CAD build for the part. Positions are in the model's coordinates, mm. Give positions to 0.01 mm unless a question says otherwise; leave off trailing zeros. Loops run counter-clockwise (first coordinate to the right, second up) from the corner with the lowest first, then second, coordinate; pieces in that order, holes last.
```python
from build123d import *

# Parameters (mm, degrees)
SKETCH1_R                = 1.5
BOSS_EXTRUDE2_DEPTH      = 1.7
BOSS_EXTRUDE3_DEPTH      = 7.3
BOSS_EXTRUDE3_DEPTH_BACK = 4.1
SKETCH2_W                = 16.43
SKETCH2_H                = 15.24


with BuildPart() as part:
    # Sketch1 → Boss-Extrude2 (new body)
    with BuildSketch(Plane(origin=(0, 0, 0), x_dir=(0, 0, -1), z_dir=(1, 0, 0))):
        with BuildLine():
            Line((-33, 66.67), (33, 66.67))
            ThreePointArc((33, 66.67), (34.414213562, 66.084213562), (35, 64.67))
            Line((35, 64.67), (35, -64.67))
            ThreePointArc((35, -64.67), (34.414213562, -66.084213562), (33, -66.67))
            Line((33, -66.67), (-33, -66.67))
            ThreePointArc((-33, -66.67), (-34.414213562, -66.084213562), (-35, -64.67))
            Line((-35, -64.67), (-35, 64.67))
            ThreePointArc((-35, 64.67), (-34.414213562, 66.084213562), (-33, 66.67))
        make_face()
        with Locations((-22.86, -37.46)):
            Circle(SKETCH1_R, mode=Mode.SUBTRACT)
        with Locations((22.86, -37.46)):
            Circle(SKETCH1_R, mode=Mode.SUBTRACT)
        with Locations((-24.13, 37.63)):
            Circle(SKETCH1_R, mode=Mode.SUBTRACT)
        with Locations((24.13, 37.63)):
            Circle(SKETCH1_R, mode=Mode.SUBTRACT)
        with Locations((8.89, -13.17)):
            Circle(SKETCH1_R, mode=Mode.SUBTRACT)
    extrude(amount=BOSS_EXTRUDE2_DEPTH)

    # Sketch2 → Boss-Extrude3 (add, two sides: drawn at the far end of the back side and taken through both)
    with BuildSketch(Plane(origin=(1.7, 0, 0), x_dir=(0, 0, -1), z_dir=(1, 0, 0)).offset(-BOSS_EXTRUDE3_DEPTH_BACK)):
        with Locations((9.225, -61.59)):
            Rectangle(SKETCH2_W, SKETCH2_H)
    extrude(amount=BOSS_EXTRUDE3_DEPTH + BOSS_EXTRUDE3_DEPTH_BACK)


solid = part.part
```
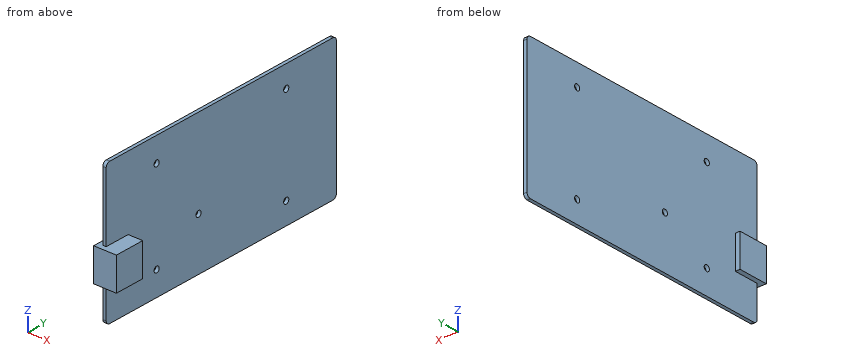
1. Probe line 1 along Y through (x, z) = (0.8, -22.86); line 2 along Y through (x, z) = (1.35, -24.13); line 3 along X through (y, z) = (39.5, 27). List the from-to ranges inside material, lowest first.
Responses:
line 1: y = -66.67 to -38.96, -35.96 to 36.83, 38.43 to 66.67
line 2: y = -66.67 to -38.26, -36.66 to 36.13, 39.13 to 66.67
line 3: x = 0 to 1.7
2. Saw through at C-C, the plane y = -13.17. List the corners of the cut face in (x, z).
Responses:
outline: (0, -35) - (1.7, -35) - (1.7, -10.39) - (0, -10.39) - close; (0, -7.39) - (1.7, -7.39) - (1.7, 35) - (0, 35) - close
3. Saw through at D-D, the plane y = -59.5. List the corners of the cut face in (x, z), and give its area (3 significant figures).
Responses:
outline: (-2.4, -17.44) - (0, -17.44) - (0, -35) - (1.7, -35) - (1.7, -17.44) - (9, -17.44) - (9, -1.01) - (1.7, -1.01) - (1.7, 35) - (0, 35) - (0, -1.01) - (-2.4, -1.01) - close
area: 278 mm2
4. Saw through at A-A, the plane y = -37.46. List the corners of the cut face in (x, z), and give its area (3 significant figures).
Responses:
outline: (0, -35) - (1.7, -35) - (1.7, -24.36) - (0, -24.36) - close; (0, -21.36) - (1.7, -21.36) - (1.7, 21.36) - (0, 21.36) - close; (0, 24.36) - (1.7, 24.36) - (1.7, 35) - (0, 35) - close
area: 109 mm2
5. Drop flat-ended pins along their axis: pin 1 (1.9 mm diameter, centred on x = 0.5, z = -24, fed in from -Y); pin 2 (5 mm diameter, centred on y = -37.46, z = -22.86, fed in from +X); pin 3 (1.8 mm diameter, centred on y = 37.63, z = 24.13, fed in from +X); pin 4 (2 mm diameter, centred on x = 6, z = -10, fed in from +Y). Give the stop position or say it passes through.
Responses:
pin 1: stops at y = -66.67
pin 2: stops at x = 1.7
pin 3: passes through
pin 4: stops at y = -53.97
6. Saw through at B-B, the plane z = -8.89. List the corners of the cut face in (x, y).
Responses:
outline: (-2.4, -69.21) - (9, -69.21) - (9, -53.97) - (1.7, -53.97) - (1.7, -14.67) - (0, -14.67) - (0, -53.97) - (-2.4, -53.97) - close; (0, -11.67) - (1.7, -11.67) - (1.7, 66.67) - (0, 66.67) - close
